CAD build for the part. Positions are in the model's coordinates, mm. Round coordinates to 2 decimals unless told otherwise and drop trailing zeros. Order: outer loops, then holes, each group sorted by start corner. A loop starts at its lowest first (then second) coordinate and runs counter-clockwise, first axis right, second up. Notation, with made-up numbers: M -9,80.25 L 6,80.25 A16 ccw 6,85.25 Z; hole C -23,4.5 d3. An arc over 180 degrees is marked long. Put each result on its own line as item: value.
```python
from build123d import *

# Parameters (mm, degrees)
BOSS_EXTRUDE1_DEPTH = 3
SKETCH2_R           = 2.1
SKETCH2_R_2         = 1.95
CUT_EXTRUDE1_DEPTH  = 4
FILLET1_R           = 2


with BuildPart() as part:
    # Sketch1 → Boss-Extrude1 (new body)
    with BuildSketch(Plane(origin=(0, 0, 0), x_dir=(1, 0, 0), z_dir=(0, 1, 0))):
        Polygon((12, 0), (52, 0), (52, 24), (-52, 24), (-52, 0), (-12, 0), (-12, -60), (12, -60), align=None)
    extrude(amount=BOSS_EXTRUDE1_DEPTH)

    # Sketch2 → Cut-Extrude1 (cut, through all)
    with BuildSketch(Plane(origin=(0, 3, 0), x_dir=(1, 0, 0), z_dir=(0, 1, 0))):
        with Locations((0, 12)):
            Circle(SKETCH2_R)
        with Locations((-8, 12)):
            Circle(SKETCH2_R)
        with Locations((0, 20)):
            Circle(SKETCH2_R_2)
        with Locations((-48, 12)):
            Circle(SKETCH2_R)
        with Locations((-48, 20)):
            Circle(SKETCH2_R)
        with Locations((-40, 12)):
            Circle(SKETCH2_R_2)
        with Locations((-40, 20)):
            Circle(SKETCH2_R)
        with Locations((-24, 12)):
            Circle(SKETCH2_R)
        with Locations((-24, 20)):
            Circle(SKETCH2_R)
        with Locations((0, -12)):
            Circle(SKETCH2_R)
        with Locations((0, -28)):
            Circle(SKETCH2_R)
        with Locations((0, -38.1)):
            Circle(SKETCH2_R_2)
        with Locations((0, -48.2)):
            Circle(SKETCH2_R)
        with Locations((0, -56.2)):
            Circle(SKETCH2_R)
        with Locations((-8, -56.2)):
            Circle(SKETCH2_R_2)
        with Locations((-8, -48.2)):
            Circle(SKETCH2_R)
        with Locations((-8, -28)):
            Circle(SKETCH2_R)
        with Locations((-8, -12)):
            Circle(SKETCH2_R)
        with Locations((0, 4)):
            Circle(SKETCH2_R_2)
        with Locations((-24, 4)):
            Circle(SKETCH2_R)
        with Locations((-40, 4)):
            Circle(SKETCH2_R)
        with Locations((-48, 4)):
            Circle(SKETCH2_R)
        with Locations((8, -56.2)):
            Circle(SKETCH2_R_2)
        with Locations((8, -48.2)):
            Circle(SKETCH2_R)
        with Locations((8, -28)):
            Circle(SKETCH2_R)
        with Locations((8, -12)):
            Circle(SKETCH2_R)
        with Locations((8, 12)):
            Circle(SKETCH2_R)
        with Locations((24, 4)):
            Circle(SKETCH2_R)
        with Locations((24, 20)):
            Circle(SKETCH2_R)
        with Locations((24, 12)):
            Circle(SKETCH2_R)
        with Locations((40, 20)):
            Circle(SKETCH2_R)
        with Locations((40, 12)):
            Circle(SKETCH2_R_2)
        with Locations((48, 12)):
            Circle(SKETCH2_R)
        with Locations((40, 4)):
            Circle(SKETCH2_R)
        with Locations((48, 4)):
            Circle(SKETCH2_R)
        with Locations((48, 20)):
            Circle(SKETCH2_R)
    extrude(amount=-CUT_EXTRUDE1_DEPTH, mode=Mode.SUBTRACT)

    # Fillet1
    fillet1_edges = [part.edges().sort_by_distance(p)[0] for p in [
        (-52, 1.5, -24),
        (52, 1.5, -24),
        (52, 1.5, 0),
        (12, 1.5, 0),
        (12, 1.5, 60),
        (-12, 1.5, 60),
        (-12, 1.5, 0),
        (-52, 1.5, 0),
    ]]
    fillet(fillet1_edges, radius=FILLET1_R)


solid = part.part
```
Item 1: Pin check, flat tips, straight feed: P1, Ø1.5, axis at x = 31.5, y = 1.5, coming from the +Z side; P2, Ø4, axis at x = 8, z = -12, coming from the -Y side. Stop position of each tip, or through.
Answers below:
P1: z = 0
P2: through
Item 2: Probe line 1 along Z through (x, y) = (-8, 2.2); line 2 along Z through (x, y) = (43, 1.15); line 3 along X through (y, z) = (1.25, 3.5). List the from-to ranges inside material, lowest first. Write a range as [from, to].
Answers below:
line 1: [-24, -14.1], [-9.9, 9.9], [14.1, 25.9], [30.1, 46.1], [50.3, 54.25], [58.15, 60]
line 2: [-24, 0]
line 3: [-12, 12]
Item 3: Band-saw the part on B-B on x = -40. Give the cut face in (y, z).
Answers below:
outline: M 0,-24 L 3,-24 L 3,-22.1 L 0,-22.1 Z; M 0,-17.9 L 3,-17.9 L 3,-13.95 L 0,-13.95 Z; M 0,-10.05 L 3,-10.05 L 3,-6.1 L 0,-6.1 Z; M 0,-1.9 L 3,-1.9 L 3,0 L 0,0 Z
Item 4: Band-saw the part on C-C on x = 8. Give the cut face in (y, z).
Answers below:
outline: M 0,-24 L 3,-24 L 3,-14.1 L 0,-14.1 Z; M 0,-9.9 L 3,-9.9 L 3,9.9 L 0,9.9 Z; M 0,14.1 L 3,14.1 L 3,25.9 L 0,25.9 Z; M 0,30.1 L 3,30.1 L 3,46.1 L 0,46.1 Z; M 0,50.3 L 3,50.3 L 3,54.25 L 0,54.25 Z; M 0,58.15 L 3,58.15 L 3,60 L 0,60 Z
Item 5: Band-saw the part on A-A on z = -4. State how many separate pieces and enclosed holes the cut face has, and give its area (3 significant figures).
Answers below:
separate pieces: 8
enclosed holes: 0
area: 225 mm²
Item 6: Mould opens along Z. For faces 1 (the flat face through (-12, 1, 30)), 2 (the cylindrical face through (38.452, 1.521, -21.419)) say: pulls with the +Z half, pulls with the -Z half, needs draft (parallel to the pull), parting line crosses it, or undercut.
Answers below:
face 1: needs draft
face 2: undercut
